```python
from build123d import *

# Parameters (mm, degrees)
SALIENTE_EXTRUIR1_DEPTH = 13.5
CROQUIS4_R              = 2.125
CORTAR_EXTRUIR1_DEPTH   = 76


with BuildPart() as part:
    # Croquis1 → Saliente-Extruir1 (new body)
    with BuildSketch(Plane.XY):
        Polygon((3.75, 0), (27, 0), (27, 55), (3.75, 55), (3.75, 58), (0, 58), (0, 55), (0, 52), (24, 52), (24, 3), (0, 3), (0, 0), (0, -3), (3.75, -3), align=None)
    extrude(amount=SALIENTE_EXTRUIR1_DEPTH)

    # Croquis4 → Cortar-Extruir1 (cut)
    with BuildSketch(Plane.XZ):
        with Locations(Location((9.25, 6.75, 0), (0, 0, 270))):
            Circle(CROQUIS4_R)
    extrude(amount=-CORTAR_EXTRUIR1_DEPTH, mode=Mode.SUBTRACT)


solid = part.part
```
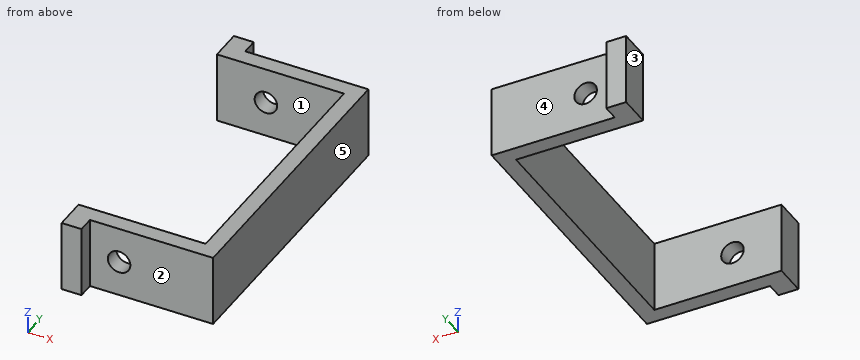
Check sheet for the modelled part. Datum: model origin and axes. Units: mm. Face numbers are marked on the shaded views. A direction names the side the tool comes from. Give positions to 0.01 mm unless a question says otherwise; leave off trailing zeros. Order: outer loops, then holes, each group sorted by start corner. A loop starts at its lowest first (then second) coordinate and runs counter-clockwise, first axis right, second up. Notation, with made-up numbers: (8.5, 18) -> (67.5, 18) arc R8 ccw to (67.5, 25) -> close; hole circle Ø2 at (64.5, 17.25). An arc over 180 degrees is marked (long way). Return JSON: item names as keys, results as strings.
1. Go/stop test with flat-tipped pins: P1, Ø1.5, axis at y = 34.5, z = 3.5, coming from the -X side; P2, Ø2, axis at x = 12.5, z = 3.5, coming from the +Y side; P3, Ø0.9, axis at y = 56, z = 4, coming from the +X side; P4, Ø2.5, axis at x = 9.25, z = 6.75, coming from the +Y side. Record where each tip stops, or that it passes through.
From the geometry:
{"P1": "x = 24", "P2": "y = 55", "P3": "x = 3.75", "P4": "through"}
2. Set-up check for the marked faces 1, 2, 3, 4 and 5: record each of +Z, -Z, +X, -X, +Y, -Y from which the full face is reachable in a straight line by a thin tool's end or side.
From the geometry:
{"face 1": "+Z, -Z, -X", "face 2": "+Z, -Z, +X, -Y", "face 3": "+Z, -Z, -X, +Y, -Y", "face 4": "+Z, -Z, +X, +Y", "face 5": "+Z, -Z, +X, +Y, -Y"}
3. Cross-section at C-C, the plane z = 6.75. Record the cut outline in (x, y) (3 decimals), plus the area to 3 significant figures.
From the geometry:
{"outline": "(0, -3) -> (3.75, -3) -> (3.75, 0) -> (7.125, 0) -> (7.125, 3) -> (0, 3) -> close; (0, 52) -> (7.125, 52) -> (7.125, 55) -> (3.75, 55) -> (3.75, 58) -> (0, 58) -> close; (11.375, 0) -> (27, 0) -> (27, 55) -> (11.375, 55) -> (11.375, 52) -> (24, 52) -> (24, 3) -> (11.375, 3) -> close", "area": "306 mm^2"}
4. Cross-section at B-B, the plane x = 18. Record the cut outline in (y, z), plus the area to 3 significant figures.
From the geometry:
{"outline": "(0, 0) -> (3, 0) -> (3, 13.5) -> (0, 13.5) -> close; (52, 0) -> (55, 0) -> (55, 13.5) -> (52, 13.5) -> close", "area": "81.0 mm^2"}
5. Cross-section at D-D, the plane y = 30.5. Record the cut outline in (x, z).
From the geometry:
{"outline": "(24, 0) -> (27, 0) -> (27, 13.5) -> (24, 13.5) -> close"}
6. Material ranges on probe 1 along Y at (x, z) = (18.25, 7.75); probe 2 along X at (y, z) = (0.95, 6.75) (3 decimals); probe 3 along Y at (x, z) = (3.5, 8.5), recorded low to high. Write a range as [from, to].
From the geometry:
{"probe 1": "[0, 3], [52, 55]", "probe 2": "[0, 7.125], [11.375, 27]", "probe 3": "[-3, 3], [52, 58]"}
7. Cross-section at A-A, the plane x = 9.25. Record the cut outline in (y, z) (3 decimals).
From the geometry:
{"outline": "(0, 0) -> (3, 0) -> (3, 4.625) -> (0, 4.625) -> close; (0, 8.875) -> (3, 8.875) -> (3, 13.5) -> (0, 13.5) -> close; (52, 0) -> (55, 0) -> (55, 4.625) -> (52, 4.625) -> close; (52, 8.875) -> (55, 8.875) -> (55, 13.5) -> (52, 13.5) -> close"}
